Here's how the part is built. I have some questions about the finished solid (model axes, mm). A direction names the side the tool comes from. Coordinates: 2 decimals unless noted, no trailing zeros. Loops run counter-clockwise (first coordinate to the right, second up) from the corner with the lowest first, then second, coordinate; pieces in that order, holes last. Notation, with made-up numbers: (51, 74.25) - (66, 74.25) arc R23 ccw to (66, 88.25) - close; hole circle Ø11 at (11.5, -31). An arc over 180 degrees is marked (long way). Use a Markdown table: item, result.
```python
from build123d import *

# Parameters (mm, degrees)
BOSS_EXTRUDE1_DEPTH = 7.5
BOSS_EXTRUDE3_DEPTH = 100
SKETCH5_R           = 6.35
CUT_EXTRUDE1_DEPTH  = 335
SKETCH6_W           = 100
SKETCH6_H           = 10
BOSS_EXTRUDE4_DEPTH = 70
SKETCH7_R           = 6.35
CUT_EXTRUDE2_DEPTH  = 322
SKETCH9_R           = 3
SKETCH9_R_2         = 5
CUT_EXTRUDE3_DEPTH  = 53
SKETCH10_R          = 6.35
BOSS_EXTRUDE5_DEPTH = 60
SKETCH11_R          = 5
CUT_EXTRUDE4_DEPTH  = 490
SKETCH12_W          = 30
SKETCH12_H          = 10
BOSS_EXTRUDE6_DEPTH = 30
SKETCH13_R          = 5
CUT_EXTRUDE5_DEPTH  = 10
SKETCH14_W          = 30
SKETCH14_H          = 10
BOSS_EXTRUDE7_DEPTH = 100
SKETCH15_R          = 5
CUT_EXTRUDE6_DEPTH  = 35


with BuildPart() as part:
    # Sketch2 → Boss-Extrude1 (new body)
    with BuildSketch(Plane.XY):
        with BuildLine():
            Line((-19.9, 200), (39.9, 200))
            Line((39.9, 200), (39.9, 164.2))
            ThreePointArc((39.9, 164.2), (44.293398282, 153.593398282), (54.9, 149.2))
            Line((54.9, 149.2), (190, 149.2))
            ThreePointArc((190, 149.2), (200.606601718, 153.593398282), (205, 164.2))
            Line((205, 164.2), (205, 200))
            Line((205, 200), (225, 200))
            Line((225, 200), (225, -200))
            Line((225, -200), (205, -200))
            Line((205, -200), (205, -164.2))
            ThreePointArc((205, -164.2), (200.606601718, -153.593398282), (190, -149.2))
            Line((190, -149.2), (54.9, -149.2))
            ThreePointArc((54.9, -149.2), (44.293398282, -153.593398282), (39.9, -164.2))
            Line((39.9, -164.2), (39.9, -200))
            Line((39.9, -200), (-19.9, -200))
            Line((-19.9, -200), (-19.9, -164.2))
            ThreePointArc((-19.9, -164.2), (-24.293398282, -153.593398282), (-34.9, -149.2))
            Line((-34.9, -149.2), (-170, -149.2))
            ThreePointArc((-170, -149.2), (-180.606601718, -153.593398282), (-185, -164.2))
            Line((-185, -164.2), (-185, -200))
            Line((-185, -200), (-225, -200))
            Line((-225, -200), (-225, 200))
            Line((-225, 200), (-185, 200))
            Line((-185, 200), (-185, 164.2))
            ThreePointArc((-185, 164.2), (-180.606601718, 153.593398282), (-170, 149.2))
            Line((-170, 149.2), (-34.9, 149.2))
            ThreePointArc((-34.9, 149.2), (-24.293398282, 153.593398282), (-19.9, 164.2))
            Line((-19.9, 164.2), (-19.9, 200))
        make_face()
    extrude(amount=BOSS_EXTRUDE1_DEPTH)

    # Sketch4 → Boss-Extrude3 (add)
    with BuildSketch(Plane.XY.offset(7.5)):
        with BuildLine():
            Line((-217.5, 192.5), (-225, 200))
            Line((-225, 200), (-185, 200))
            Line((-185, 200), (-185, 164.2))
            ThreePointArc((-185, 164.2), (-180.606601718, 153.593398282), (-170, 149.2))
            Line((-170, 149.2), (-34.9, 149.2))
            ThreePointArc((-34.9, 149.2), (-24.293398282, 153.593398282), (-19.9, 164.2))
            Line((-19.9, 164.2), (-19.9, 200))
            Line((-19.9, 200), (39.9, 200))
            Line((39.9, 200), (39.9, 164.2))
            ThreePointArc((39.9, 164.2), (44.293398282, 153.593398282), (54.9, 149.2))
            Line((54.9, 149.2), (190, 149.2))
            ThreePointArc((190, 149.2), (200.606601718, 153.593398282), (205, 164.2))
            Line((205, 164.2), (205, 200))
            Line((205, 200), (225, 200))
            Line((225, 200), (225, -200))
            Line((225, -200), (205, -200))
            Line((205, -200), (205, -164.2))
            ThreePointArc((205, -164.2), (200.606601718, -153.593398282), (190, -149.2))
            Line((190, -149.2), (54.9, -149.2))
            ThreePointArc((54.9, -149.2), (44.293398282, -153.593398282), (39.9, -164.2))
            Line((39.9, -164.2), (39.9, -200))
            Line((39.9, -200), (-19.9, -200))
            Line((-19.9, -200), (-19.9, -164.2))
            ThreePointArc((-19.9, -164.2), (-24.293398282, -153.593398282), (-34.9, -149.2))
            Line((-34.9, -149.2), (-170, -149.2))
            ThreePointArc((-170, -149.2), (-180.606601718, -153.593398282), (-185, -164.2))
            Line((-185, -164.2), (-185, -200))
            Line((-185, -200), (-225, -200))
            Line((-225, -200), (-217.5, -192.5))
            Line((-217.5, -192.5), (-192.5, -192.5))
            Line((-192.5, -192.5), (-192.5, -164.2))
            ThreePointArc((-192.5, -164.2), (-185.909902577, -148.290097423), (-170, -141.7))
            Line((-170, -141.7), (-34.9, -141.7))
            ThreePointArc((-34.9, -141.7), (-18.990097423, -148.290097423), (-12.4, -164.2))
            Line((-12.4, -164.2), (-12.4, -192.5))
            Line((-12.4, -192.5), (32.4, -192.5))
            Line((32.4, -192.5), (32.4, -164.2))
            ThreePointArc((32.4, -164.2), (38.990097423, -148.290097423), (54.9, -141.7))
            Line((54.9, -141.7), (190, -141.7))
            ThreePointArc((190, -141.7), (205.909902577, -148.290097423), (212.5, -164.2))
            Line((212.5, -164.2), (212.5, -192.5))
            Line((212.5, -192.5), (217.5, -192.5))
            Line((217.5, -192.5), (217.5, 192.5))
            Line((217.5, 192.5), (212.5, 192.5))
            Line((212.5, 192.5), (212.5, 164.2))
            ThreePointArc((212.5, 164.2), (205.909902577, 148.290097423), (190, 141.7))
            Line((190, 141.7), (54.9, 141.7))
            ThreePointArc((54.9, 141.7), (38.990097423, 148.290097423), (32.4, 164.2))
            Line((32.4, 164.2), (32.4, 192.5))
            Line((32.4, 192.5), (-12.4, 192.5))
            Line((-12.4, 192.5), (-12.4, 164.2))
            ThreePointArc((-12.4, 164.2), (-18.990097423, 148.290097423), (-34.9, 141.7))
            Line((-34.9, 141.7), (-170, 141.7))
            ThreePointArc((-170, 141.7), (-185.909902577, 148.290097423), (-192.5, 164.2))
            Line((-192.5, 164.2), (-192.5, 192.5))
            Line((-192.5, 192.5), (-217.5, 192.5))
        make_face()
    extrude(amount=BOSS_EXTRUDE3_DEPTH)

    # Sketch5 → Cut-Extrude1 (cut)
    with BuildSketch(Plane.XZ.offset(149.2)):
        with Locations((-102.45, 40)):
            Circle(SKETCH5_R)
        with Locations((122.45, 40)):
            Circle(SKETCH5_R)
    extrude(amount=-CUT_EXTRUDE1_DEPTH, mode=Mode.SUBTRACT)

    # Sketch6 → Boss-Extrude4 (add)
    with BuildSketch(Plane.XY.offset(7.5)):
        with Locations((87.5, 66.7)):
            Rectangle(SKETCH6_W, SKETCH6_H)
        with Locations((87.5, -66.7)):
            Rectangle(SKETCH6_W, SKETCH6_H)
    extrude(amount=BOSS_EXTRUDE4_DEPTH)

    # Sketch7 → Cut-Extrude2 (cut)
    with BuildSketch(Plane.XZ.offset(149.2)):
        with Locations((122.45, 40)):
            Circle(SKETCH7_R)
    extrude(amount=-CUT_EXTRUDE2_DEPTH, mode=Mode.SUBTRACT)

    # Sketch9 → Cut-Extrude3 (cut)
    with BuildSketch(Plane.XZ.offset(-61.7)):
        with Locations((72.5, 15.5)):
            Circle(SKETCH9_R)
        with Locations((51.282377607, 52.25)):
            Circle(SKETCH9_R)
        with Locations((93.717622393, 52.25)):
            Circle(SKETCH9_R)
        with Locations((72.5, 40)):
            Circle(SKETCH9_R_2)
    cut_extrude3 = extrude(amount=-CUT_EXTRUDE3_DEPTH, mode=Mode.SUBTRACT)

    # Mirror1: Cut-Extrude3 across plane
    add(cut_extrude3.mirror(Plane.ZX), mode=Mode.SUBTRACT)

    # Sketch10 → Boss-Extrude5 (add)
    with BuildSketch(Plane(origin=(0, -141.7, 0), x_dir=(1, 0, 0), z_dir=(0, 1, 0))):
        with Locations((-102.45, -40)):
            Circle(SKETCH10_R)
    boss_extrude5 = extrude(amount=-BOSS_EXTRUDE5_DEPTH)

    # Mirror2: Boss-Extrude5 across plane
    add(boss_extrude5.mirror(Plane.ZX))

    # Sketch11 → Cut-Extrude4 (cut)
    with BuildSketch(Plane.XZ.offset(200)):
        with Locations((-205, 77.5)):
            Circle(SKETCH11_R)
        with Locations((-205, 30)):
            Circle(SKETCH11_R)
    extrude(amount=-CUT_EXTRUDE4_DEPTH, mode=Mode.SUBTRACT)

    # Sketch12 → Boss-Extrude6 (add)
    with BuildSketch(Plane.XY.offset(7.5)):
        with Locations((-17.4, 126.7)):
            Rectangle(SKETCH12_W, SKETCH12_H)
    boss_extrude6 = extrude(amount=BOSS_EXTRUDE6_DEPTH)

    # Sketch13 → Cut-Extrude5 (cut)
    with BuildSketch(Plane.XZ.offset(-121.7)):
        with Locations((-17.4, 22.5)):
            Circle(SKETCH13_R)
    cut_extrude5 = extrude(amount=-CUT_EXTRUDE5_DEPTH, mode=Mode.SUBTRACT)

    # Mirror3: Boss-Extrude6, Cut-Extrude5 across plane
    add(boss_extrude6.mirror(Plane.ZX))
    add(cut_extrude5.mirror(Plane.ZX), mode=Mode.SUBTRACT)

    # Sketch14 → Boss-Extrude7 (add)
    with BuildSketch(Plane.XY.offset(7.5)):
        with Locations((-210, 145)):
            Rectangle(SKETCH14_W, SKETCH14_H)
    boss_extrude7 = extrude(amount=BOSS_EXTRUDE7_DEPTH)

    # Sketch15 → Cut-Extrude6 (cut)
    with BuildSketch(Plane.XZ.offset(-140)):
        with Locations((-210, 77.5)):
            Circle(SKETCH15_R)
        with Locations((-210, 57.5)):
            Circle(SKETCH15_R)
        with Locations((-210, 37.5)):
            Circle(SKETCH15_R)
    cut_extrude6 = extrude(amount=-CUT_EXTRUDE6_DEPTH, mode=Mode.SUBTRACT)

    # Mirror4: Boss-Extrude7, Cut-Extrude6 across plane
    add(boss_extrude7.mirror(Plane.ZX))
    add(cut_extrude6.mirror(Plane.ZX), mode=Mode.SUBTRACT)


solid = part.part
```
Q1. I want a section at B-B, the plane y = 86.5. Write out the boundary of the cut face in (x, z).
Check values:
| item | result |
|---|---|
| outline | (-225, 0) - (225, 0) - (225, 107.5) - (217.5, 107.5) - (217.5, 7.5) - (-225, 7.5) - close |
Q2. Which directions (+Z, -Z, +X, -X, +Y, -Y) give clear straight access to the entire face, cutting with the end or side of a thin tool? Please do faces 1 (the face through (137.5, 67, 42)), 2 (the face through (-200.23, -196.3, 31.5)), 3 (the face through (-205, -192.5, 57)).
Check values:
| item | result |
|---|---|
| face 1 | +Z |
| face 2 | -Y |
| face 3 | +Z, -X |
Q3. Please list where these lines run through material, in increasing order: L1, parallel to X at y = -66, z = 15.5; L2, parallel to Y at x = -204.5, z = 88; L3, parallel to X at y = -64, z = 52.25. Write a range as from..to.
Check values:
| item | result |
|---|---|
| L1 | 37.5..69.5, 75.5..137.5, 217.5..225 |
| L2 | -200..-192.5, -150..-140, 140..150, 192.5..200 |
| L3 | 37.5..48.28, 54.28..90.72, 96.72..137.5, 217.5..225 |
Q4. I want a section at C-C, the plane x = 165.5. Write out the boundary of the cut face in (y, z).
Check values:
| item | result |
|---|---|
| outline | (-149.2, 0) - (149.2, 0) - (149.2, 107.5) - (141.7, 107.5) - (141.7, 7.5) - (-141.7, 7.5) - (-141.7, 107.5) - (-149.2, 107.5) - close |
Q5. Will these pins go through, and if not, where does the flat tip stop? P1, Ø14.5, axis at x = 122.45, z = 40, coming from the -Y side; P2, Ø8, axis at x = -210, z = 77.5, coming from the +Y side; P3, Ø4, axis at x = -140, z = 55.5, coming from the +Y side.
Check values:
| item | result |
|---|---|
| P1 | y = -149.2 |
| P2 | y = 200 |
| P3 | y = 149.2 |
Q6. I want a section at A-A, the plane x = -102.45. Write out the boundary of the cut face in (y, z).
Check values:
| item | result |
|---|---|
| outline | (-201.7, 33.65) - (-149.2, 33.65) - (-149.2, 0) - (149.2, 0) - (149.2, 33.65) - (201.7, 33.65) - (201.7, 46.35) - (149.2, 46.35) - (149.2, 107.5) - (141.7, 107.5) - (141.7, 7.5) - (-141.7, 7.5) - (-141.7, 107.5) - (-149.2, 107.5) - (-149.2, 46.35) - (-201.7, 46.35) - close |
Q7. If we mould it in two halves opening along Z, with no side actions, what happens to faces 4 (the face through (206.084, 148.466, 56.8)), 5 (the face through (-205.23, -144.93, 59)), 6 (the face through (-103.277, 175.082, 33.704))? For each: pulls with the +Z half, pulls with the -Z half, needs draft (parallel to the pull), parting line crosses it, or undercut.
Check values:
| item | result |
|---|---|
| face 4 | needs draft |
| face 5 | undercut |
| face 6 | parting line crosses it |
